```python
from build123d import *

# Parameters (mm, degrees)
F0_R        = 8
F1_DEPTH    = 20
F2_W        = 10
F2_H        = 20.4895668926
F3_DEPTH    = 10
F4_W        = 20
F4_H        = 4
F5_DEPTH    = 50
F6_T1_DEPTH = 37.4899959968
F7_R        = 2
F9_DEPTH    = 50
F10_R       = 1
F11_DEPTH   = 25


# Not quite as in the source:
# - a fillet or chamfer that OpenCascade refuses, or shapes differently, is made with other operations: its cross-section is extruded or revolved along the edge and cut away or added


with BuildPart() as f1:
    # F0 (on Front) → F1 (new body)
    with BuildSketch(Plane.XZ):
        Circle(F0_R)
    extrude(amount=F1_DEPTH)

    # F2 (on Front) → F3 (cut)
    with BuildSketch(Plane.XZ):
        Rectangle(F2_W, F2_H)
    extrude(amount=F3_DEPTH, mode=Mode.SUBTRACT)

    # F4 (on Right) → F5 (cut, symmetric)
    with BuildSketch(Plane.YZ):
        with Locations((-19.8148275974, 0)):
            Rectangle(F4_W, F4_H)
    extrude(amount=F5_DEPTH, both=True, mode=Mode.SUBTRACT)

    # F6: fillet of radius 5 on 2 edges, made by hand

    # F6_s2 → F6_t1 (cut)
    with BuildSketch(Plane.XY.offset(-18.7449979984)):
        with BuildLine():
            ThreePointArc((10, 0), (6.4644660941, -1.4644660941), (5, -5))
            Line((5, -5), (5, 0))
            Line((5, 0), (10, 0))
        make_face()
        with BuildLine():
            ThreePointArc((-5, -5), (-6.4644660941, -1.4644660941), (-10, 0))
            Line((-10, 0), (-5, 0))
            Line((-5, 0), (-5, -5))
        make_face()
    extrude(amount=F6_T1_DEPTH, mode=Mode.SUBTRACT)

    # F7
    f7_edges = [f1.edges().sort_by_distance(p)[0] for p in [
        (0, -20, -2),
        (0, -20, 2),
    ]]
    fillet(f7_edges, radius=F7_R)

    # F8 (on face) → F9 (cut, symmetric)
    with BuildSketch(Plane.YZ.offset(-5)):
        with BuildLine():
            Line((-5, -1), (-5, 1))
            ThreePointArc((-5, 1), (-6, 0), (-5, -1))
        make_face()
        with BuildLine():
            ThreePointArc((-5, -1), (-4.2928932188, -0.7071067812), (-4, 0))
            ThreePointArc((-4, 0), (-4.2928932188, 0.7071067812), (-5, 1))
            Line((-5, 1), (-5, -1))
        make_face()
    extrude(amount=F9_DEPTH, both=True, mode=Mode.SUBTRACT)

    # F10 (on Top) → F11 (cut, symmetric)
    with BuildSketch(Plane.XY):
        with Locations((0, -16)):
            Circle(F10_R)
    extrude(amount=F11_DEPTH, both=True, mode=Mode.SUBTRACT)


solid = f1.part
```
Source: CAD feature listing. Evaluate the final solid. Frame: model axes, mm. A direction names the side the tool comes from. Round coordinates to 2 decimals unless told otherwise and drop trailing zeros. Loops run counter-clockwise (first coordinate to the right, second up) from the corner with the lowest first, then second, coordinate; pieces in that order, holes last. Notation, with made-up numbers: M -28,82.25 L -10,82.25 A17 cw -10,111.25 Z; hole C -28.5,88.25 d6. An arc over 180 degrees is marked long. Use a Markdown table: item, result. Add a question column.
1. Reachability of faces 5 (the flat face through (0, -14, -2)), 6 (the flat face through (0, -20, 6)), 7 (the flat face through (5, -7, 0)) from +Z, -Z, +X, -X, +Y, -Y: full face, straight path, thin tool, end or side. Return the list, or none.
2. Section query D-D on z = -5.5. Return the cut outline in (x, y).
3. Mould query, pull axis Y, two halves, no side actions, for faces 1 (the cylindrical face through (0, -17, -5)), 2 (the flat face through (-5, -7, 0)), 3 (the flat face through (0, -10, 5)), 4 (the flat face through (0, -20, -6)). Classes: pulls with the +Y half, pulls with the -Y half, needs draft (parallel to the pull), parting line crosses it, or undercut.
4. Section query C-C on x = 4.25. Return the cut outline in (y, z).
5. Line query: line 1 (Y direction, x = 0, z = -6.5); line 2 (X direction, y = -16, z = -5) (3 decimals); line 3 (Z direction, x = 0, y = -12.75). Output: solid intervals per line, ascending.
6. Section query B-B on y = -13.75. Return the cut outline in (x, z).
7. Section query A-A on x = 0. Return the cut outline in (y, z), then the cut area to 3 significant figures.
8. Contact query for flat-ended pins moving along their axis: P1, Ø1, axis at y = -15, z = 4.5, coming from the -X side; P2, Ø1.8, axis at x = 0.5, z = 4.5, coming from the +Y side; P3, Ø2, axis at x = -5.5, y = -16, coming from the +Z side. Output: stop coordinate, or through.
Reported:
| question | item | result |
|---|---|---|
| 1 | face 5 | +X, -X, -Y |
| 1 | face 6 | +Z, -Z, +X, -X, -Y |
| 1 | face 7 | +Z, -Z, +Y |
| 2 | outline | M -5.81,-20 L 5.81,-20 L 5.81,-2.27 A5 ccw 5,-5 L 5,-10 L -5,-10 L -5,-5 A5 ccw -5.81,-2.27 Z; hole C 0,-16 d2 |
| 3 | face 1 | undercut |
| 3 | face 2 | needs draft |
| 3 | face 3 | pulls with the +Y half |
| 3 | face 4 | pulls with the -Y half |
| 4 | outline | M -20,-6.78 L -10,-6.78 L -10,-2 L -18,-2 A2 ccw -20,-4 Z; M -20,4 A2 ccw -18,2 L -10,2 L -10,6.78 L -20,6.78 Z |
| 5 | line 1 | y = -20 to -17, -15 to -10 |
| 5 | line 2 | x = -6.245 to -1, 1 to 6.245 |
| 5 | line 3 | z = -8 to -2, 2 to 8 |
| 6 | outline | M -7.75,-2 A8 ccw 7.75,-2 Z; M -7.75,2 L 7.75,2 A8 ccw Z |
| 7 | outline | M -20,-8 L -17,-8 L -17,-2 L -18,-2 A2 ccw -20,-4 Z; M -20,4 A2 ccw -18,2 L -17,2 L -17,8 L -20,8 Z; M -15,-8 L -10,-8 L -10,-2 L -15,-2 Z; M -15,2 L -10,2 L -10,8 L -15,8 Z |
| 7 | area | 94.3 mm² |
| 8 | P1 | stops at x = -6.93 |
| 8 | P2 | stops at y = -10 |
| 8 | P3 | stops at z = 6.61 |
